from build123d import *

# Parameters (mm, degrees)
F0_W     = 25.4
F0_H     = 12.7
F1_DEPTH = 50.8
F3_DEPTH = 12.7
F5_DEPTH = 38.1
F7_DEPTH = 76.201


with BuildPart() as f1:
    # F0 (on Top) → F1 (new body)
    with BuildSketch(Plane.XY):
        with Locations((12.7, 44.45)):
            Rectangle(F0_W, F0_H)
        Polygon((25.4, 38.1), (38.1, 38.1), (50.8, 38.1), (50.8, 50.8), (25.4, 50.8), align=None)
        with Locations((63.5, 44.45)):
            Rectangle(F0_W, F0_H)
    extrude(amount=F1_DEPTH)

    # F2 (on face) → F3 (cut)
    with BuildSketch(Plane(origin=(0, 50.8, 0), x_dir=(-1, 0, 0), z_dir=(0, 1, 0))):
        Polygon((-76.2, 25.4), (-50.8, 50.8), (-76.2, 50.8), align=None)
        Polygon((-25.4, 50.8), (0, 25.4), (0, 50.8), align=None)
    extrude(amount=-F3_DEPTH, mode=Mode.SUBTRACT)

    # F4 (on face) → F5 (join)
    with BuildSketch(Plane.XZ.offset(-38.1)):
        Polygon((38.1, 38.1), (0, 0), (19.05, 0), (19.05, 12.7), (57.15, 12.7), (57.15, 0), (76.2, 0), align=None)
    extrude(amount=F5_DEPTH)

    # F6 (on face) → F7 (cut, through all)
    with BuildSketch(Plane.YZ.offset(76.2)):
        Polygon((38.1, 38.1), (0, 38.1), (0, 0), align=None)
    extrude(amount=-F7_DEPTH, mode=Mode.SUBTRACT)


solid = f1.part
The listing builds one solid part. Answer for the finished solid, in the listing's coordinates (mm). A direction names the side the tool comes from. Give positions to 0.01 mm unless a question says otherwise; leave off trailing zeros. Order: outer loops, then holes, each group sorted by start corner. A loop starts at its lowest first (then second) coordinate and runs counter-clockwise, first axis right, second up. Notation, with made-up numbers: (20, -27) - (34, -27) arc R24 cw to (34, 4) - close; hole circle Ø9 at (-14.5, 63.5). An arc over 180 degrees is marked (long way). Use one line per item in the form item = value.
1) Find section B-B on z = 16. Determine the outline of the cut face in (x, y), and give its area (3 significant figures).
Verdict:
outline = (0, 38.1) - (16, 38.1) - (16, 16) - (60.2, 16) - (60.2, 38.1) - (76.2, 38.1) - (76.2, 50.8) - (0, 50.8) - close
area = 1,940 mm^2
2) Each of these flat-tipped pins is pushed along its axis until it touches: pin 1 (6.5 mm diameter, centred on x = 29.5, z = 8, fed in from -Y); pin 2 (10 mm diameter, centred on y = 25.5, z = 6.5, fed in from -X); pin 3 (12 mm diameter, centred on y = 33, z = 45.5, fed in from +X); pin 4 (10 mm diameter, centred on y = 28, z = 40, fed in from -X). Where does it stop, or does it pass through?
Verdict:
pin_1 = 38.1
pin_2 = 1.5
pin_3 = 59.26
pin_4 = through
3) Consider probe 1 along Y at (x, z) = (9, 29.5); probe 2 along X at (y, z) = (37, 8); probe 3 along Y at (x, z) = (36, 32.5). Determine where each line is inside the solid, lowest interval first. Write a range as [from, to].
Verdict:
probe_1 = [38.1, 50.8]
probe_2 = [8, 19.05], [57.15, 68.2]
probe_3 = [32.5, 50.8]
4) Find section C-C on y = 3. Determine the outline of the cut face in (x, z), and give its area (3 significant figures).
Verdict:
outline = (0, 0) - (19.05, 0) - (19.05, 3) - (3, 3) - close; (57.15, 0) - (76.2, 0) - (73.2, 3) - (57.15, 3) - close
area = 105 mm^2
5) The mould has two halves that part along X. Classify faces 6 (the flat face through (76.2, 44, 13)), 7 (the flat face through (12.9, 44.5, 38.3)), 8 (the flat face through (57.15, 24, 6)), 9 (the flat face through (38, 43, 0)): released by +X, released by -X, zero draft, split by the parting line, or undercut.
Verdict:
face_6 = released by +X
face_7 = released by -X
face_8 = undercut
face_9 = zero draft
6) For faces 1 (the flat face through (39, 50.8, 19)), 2 (the flat face through (29, 38.1, 31)), 3 (the flat face through (11, 28, 11)), 4 (the flat face through (19.05, 24, 6)), 5 (the flat face through (61.7, 23.6, 14.5)), determine the directions among +Z, -Z, +X, -X, +Y, -Y from which every point of the face is accessible in a straight line to the end or side of a thin tool.
Verdict:
face_1 = +Z, -Z, +X, -X, +Y
face_2 = +Z, -Y
face_3 = +Z, -X, -Y
face_4 = -Z, -Y
face_5 = +Z, +X, -Y
7) Find section A-A on y = 14. Determine the outline of the cut face in (x, z).
Verdict:
outline = (0, 0) - (19.05, 0) - (19.05, 12.7) - (57.15, 12.7) - (57.15, 0) - (76.2, 0) - (62.2, 14) - (14, 14) - close
8) Find section D-D on x = 15.5. Determine the outline of the cut face in (y, z), and give its area (3 significant figures).
Verdict:
outline = (0, 0) - (50.8, 0) - (50.8, 40.9) - (38.1, 40.9) - (38.1, 15.5) - (15.5, 15.5) - close
area = 990 mm^2
